Study the drawing (mm; zero at the part's minimum x, y, z) and answer. Coordinates: 2 decimals unless noted, no trailing zeros. Order: outer loops, then holes, each group sorted by start corner. A loop starts at its lowest first (then second) coordinate and runs counter-clockwise, first axis right, second up.
1. Flat-ended cylindrical pins translate along their axes: pin 1 Ø2 at (y, z) = (3.5, 42) entering from -X; pin 2 Ø3 at (x, y) = (64.5, 1.5) entering from -Z. Find the tip coordinate at first contact, or state that the pin passes through.
2. The part is cut by section C-C, the plane y = 3.75. Give the vertices of the cut face in (x, z).
3. The part is cut by section A-A, the plane x = 38.1. Give the vertices of the cut face in (y, z), then the cut area to 3 significant figures.
4. The part is cut by section B-B, the plane z = 76.2. Give the vertices of the cut face in (x, y).
5. Find the intervals of material crossed by probe 1 along X at (y, z) = (3.5, 74.5); probe 2 along Z at (x, y) = (63.5, 3.25); probe 3 along Z at (x, y) = (16, 6), in increasing order.
6. The part is cut by section D-D, the plane z = 19.05. Give the vertices of the cut face in (x, y).
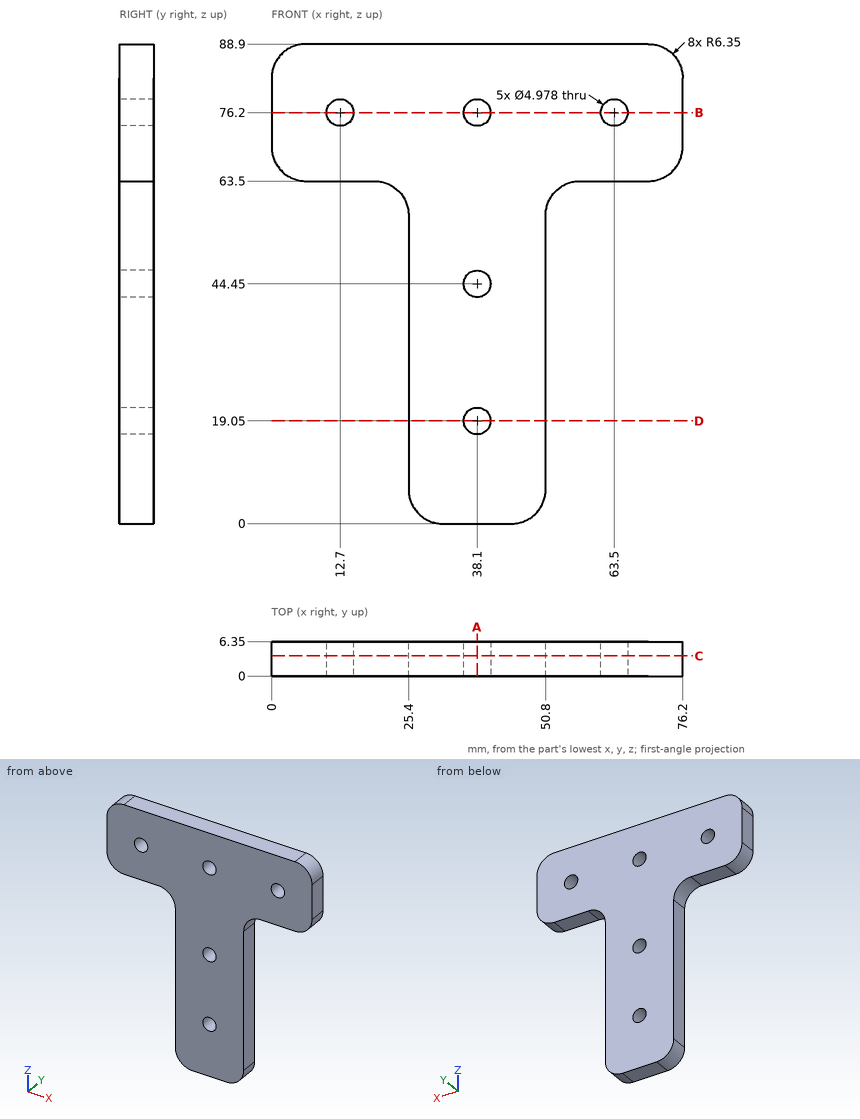
Geometry says:
1. pin 1: stops at x = 25.4
1. pin 2: stops at z = 63.5
2. outline: (0, 69.85) arc R6.35 ccw to (6.35, 63.5) - (19.05, 63.5) arc R6.35 cw to (25.4, 57.15) - (25.4, 6.35) arc R6.35 ccw to (31.75, 0) - (44.45, 0) arc R6.35 ccw to (50.8, 6.35) - (50.8, 57.15) arc R6.35 cw to (57.15, 63.5) - (69.85, 63.5) arc R6.35 ccw to (76.2, 69.85) - (76.2, 82.55) arc R6.35 ccw to (69.85, 88.9) - (6.35, 88.9) arc R6.35 ccw to (0, 82.55) - close; hole circle Ø4.98 at (12.7, 76.2); hole circle Ø4.98 at (38.1, 19.05); hole circle Ø4.98 at (38.1, 44.45); hole circle Ø4.98 at (38.1, 76.2); hole circle Ø4.98 at (63.5, 76.2)
3. outline: (0, 0) - (6.35, 0) - (6.35, 16.56) - (0, 16.56) - close; (0, 21.54) - (6.35, 21.54) - (6.35, 41.96) - (0, 41.96) - close; (0, 46.94) - (6.35, 46.94) - (6.35, 73.71) - (0, 73.71) - close; (0, 78.69) - (6.35, 78.69) - (6.35, 88.9) - (0, 88.9) - close
3. area: 470 mm2
4. outline: (0, 0) - (10.21, 0) - (10.21, 6.35) - (0, 6.35) - close; (15.19, 0) - (35.61, 0) - (35.61, 6.35) - (15.19, 6.35) - close; (40.59, 0) - (61.01, 0) - (61.01, 6.35) - (40.59, 6.35) - close; (65.99, 0) - (76.2, 0) - (76.2, 6.35) - (65.99, 6.35) - close
5. probe 1: x = 0 to 10.88, 14.52 to 36.28, 39.92 to 61.68, 65.32 to 76.2
5. probe 2: z = 63.5 to 73.71, 78.69 to 88.9
5. probe 3: z = 63.5 to 88.9
6. outline: (25.4, 0) - (35.61, 0) - (35.61, 6.35) - (25.4, 6.35) - close; (40.59, 0) - (50.8, 0) - (50.8, 6.35) - (40.59, 6.35) - close
